from build123d import *

# Parameters (mm, degrees)
SKETCH1_R           = 2
BOSS_EXTRUDE1_DEPTH = 5
SKETCH3_R           = 2
BOSS_EXTRUDE2_DEPTH = 10


with BuildPart() as part:
    # Sketch1 → Boss-Extrude1 (new body)
    with BuildSketch(Plane(origin=(0, 0, 0), x_dir=(1, 0, 0), z_dir=(0, 1, 0))):
        with BuildLine():
            Line((0, 0), (25, 0))
            ThreePointArc((25, 0), (32.5, 7.5), (25, 15))
            Line((25, 15), (0, 15))
            ThreePointArc((0, 15), (-7.5, 7.5), (0, 0))
        make_face()
        with Locations((0, 7.5)):
            Circle(SKETCH1_R, mode=Mode.SUBTRACT)
        with Locations((25, 7.5)):
            Circle(SKETCH1_R, mode=Mode.SUBTRACT)
    extrude(amount=BOSS_EXTRUDE1_DEPTH)

    # Sketch3 → Boss-Extrude2 (add)
    with BuildSketch(Plane(origin=(0, 0, -15), x_dir=(-1, 0, 0), z_dir=(0, 0, -1))):
        with BuildLine():
            Line((-20, 5), (-5, 5))
            Line((-5, 5), (-5, 30))
            ThreePointArc((-5, 30), (-12.5, 37.5), (-20, 30))
            Line((-20, 30), (-20, 5))
        make_face()
        with Locations((-12.5, 30)):
            Circle(SKETCH3_R, mode=Mode.SUBTRACT)
    extrude(amount=-BOSS_EXTRUDE2_DEPTH)


solid = part.part
The listing builds one solid part. Answer for the finished solid, in the listing's coordinates (mm). A direction names the side the tool comes from. Give positions to 0.01 mm unless a question says otherwise; leave off trailing zeros. Write each loop counter-clockwise with the first axis right and the second up, starting at its lowest first coordinate (ties: lowest second). Pieces come first, ordered by that corner, then holes.
Item 1: Section C-C, the plane z = -13.5 is taken. Write down the section's boundary in (x, y), plus the area to 3 significant figures.
Item 2: Determine the mould class of faces 4 (the cylindrical face through (12.934, 28.048, -10.07)), 5 (the cylindrical face through (23.526, 2.465, -8.852)), 6 (the cylindrical face through (12.34, 37.5, -10.07)) for opening direction Y: released by +Y, released by -Y, zero draft, split by the parting line, or undercut.
Item 3: Section D-D, the plane x = 12.5 is taken. Write down the section's boundary in (y, z), plus the area to 3 significant figures.
Item 4: Flat-ended cylindrical pins translate along their axes: P1, Ø3, axis at x = 28, z = -7, coming from the +Y side; P2, Ø3, axis at y = 17, z = -12, coming from the +X side; P3, Ø2.5, axis at x = 12.5, y = 30, coming from the -Z side; P4, Ø8, axis at y = 13.5, z = -7.5, coming from the -X side. Find the tip coordinate at first contact, or state that the pin passes through.
Item 5: Section B-B, the plane y = 3 is taken. Write down the section's boundary in (x, z), plus the area to 3 significant figures.
Item 6: Find the intervals of material crossed by line 1 along X through (y, z) = (1.6, -7.5); line 2 along Z through (x, y) = (25, 1.95); line 3 along Y through (x, z) = (12.5, -11.75), in increasing order.
Item 7: Which of the six approach directions +Z, -Z, +X, -X, +Y, -Y give full straight-line access (tool end or side, diameter ignored) to faces 1 (the flat face through (20, 18, -10)), 2 (the flat face through (13, 21, -5)), 3 (the flat face through (5, 17, -10))?
Item 8: Section A-A, the plane z = -7.5 is taken. Write down the section's boundary in (x, y).
Completed:
1. outline: (-4.5, 0) - (29.5, 0) - (29.5, 5) - (20, 5) - (20, 30) arc R7.5 ccw to (5, 30) - (5, 5) - (-4.5, 5) - close; hole circle Ø4 at (12.5, 30)
1. area: 621 mm2
2. face 4: undercut
2. face 5: zero draft
2. face 6: released by +Y
3. outline: (0, -15) - (28, -15) - (28, -5) - (5, -5) - (5, 0) - (0, 0) - close; (32, -15) - (37.5, -15) - (37.5, -5) - (32, -5) - close
3. area: 360 mm2
4. P1: stops at y = 5
4. P2: stops at x = 20
4. P3: passes through
4. P4: stops at x = 5
5. outline: (0, -15) - (25, -15) arc R7.5 ccw to (25, 0) - (0, 0) arc R7.5 ccw to start; hole circle Ø4 at (0, -7.5); hole circle Ø4 at (25, -7.5)
5. area: 527 mm2
6. line 1: x = -7.5 to -2, 2 to 23, 27 to 32.5
6. line 2: z = -15 to -9.5, -5.5 to 0
6. line 3: y = 0 to 28, 32 to 37.5
7. face 1: +Z, -Z, +X, +Y
7. face 2: +Z, +X, -X, +Y
7. face 3: +Z, -Z, -X, +Y
8. outline: (-7.5, 0) - (-2, 0) - (-2, 5) - (-7.5, 5) - close; (2, 0) - (23, 0) - (23, 5) - (20, 5) - (20, 30) arc R7.5 ccw to (5, 30) - (5, 5) - (2, 5) - close; (27, 0) - (32.5, 0) - (32.5, 5) - (27, 5) - close; hole circle Ø4 at (12.5, 30)
